Input: part model. Units: mm. Frame: model coordinates. A direction names the side the tool comes from. Give positions to 0.01 mm unless a question says otherwise; leave off trailing zeros. Loops run counter-clockwise (first coordinate to the right, second up) from the corner with the lowest first, then second, coordinate; pieces in that order, holes last. Notation, with made-up numbers: (-24.5, 88) - (-0.5, 88) arc R13 cw to (-0.5, 92) - close; hole circle Ø6 at (-4.5, 54). An arc over 180 degrees is marked (long way). One line per item, written item: value.
Autodesk Inventor part; units mm, degrees
ref_plane "YZ Plane" through (0, 0, 0) normal (1, 0, 0) x (0, 1, 0)
ref_plane "XZ Plane" through (0, 0, 0) normal (0, 1, 0) x (-1, 0, 0)
ref_plane "XY Plane" through (0, 0, 0) normal (0, 0, 1) x (1, 0, 0)
sketch "スケッチ1" plane through (0, 0, 0) normal (0, 0, 1) x (1, 0, 0)
  line L0 (62.5, -15) -> (-62.5, -15)
  line L1 (-62.5, -15) -> (-62.5, 15)
  line L2 (-62.5, 15) -> (62.5, 15)
  line L3 (62.5, 15) -> (62.5, -15)
  line L4 (62.5, -15) -> (-62.5, 15) construction
  line L5 (-62.5, -15) -> (62.5, 15) construction
  point P0 (0, 0)
  dimension "d0" = 30
  dimension "d1" = 125
extrude "押し出し1" add sketch "スケッチ1" along normal blind 34
sketch "スケッチ2" plane through (-62.5, 15, 0) normal (0, 1, 0) x (1, 0, 0)
  line L0 (125, 0) -> (95, 0)
  line L1 (95, 0) -> (95, -6)
  line L2 (95, -6) -> (125, -6)
  line L3 (125, -6) -> (125, 0)
  point P0 (62.5, 0)
  dimension "d4" = 30
  dimension "d5" = 6
extrude "押し出し2" cut sketch "スケッチ2" against normal blind 34
sketch "スケッチ3" plane through (-62.5, 15, 34) normal (0, 1, 0) x (1, 0, 0)
  line L0 (0, 0) -> (125, 0)
  line L1 (90, 0) -> (5, 0)
  line L2 (5, 0) -> (5, 21)
  line L3 (5, 21) -> (90, 21)
  line L4 (90, 21) -> (90, 0)
  line L5 (0, 34) -> (0, 0)
  line L6 (95, 28) -> (95, 34)
  line L7 (95, 34) -> (0, 34)
  point P0 (62.5, 34)
  point P1 (5, 0)
  dimension "d8" = 5
  dimension "d9" = 5
  dimension "d10" = 13
extrude "押し出し3" cut sketch "スケッチ3" against normal blind 34
sketch "スケッチ4" plane through (-62.5, 15, 34) normal (0, 1, 0) x (1, 0, 0)
  line L0 (90, 21) -> (90, 0)
  line L1 (125, 0) -> (90, 0)
  line L2 (125, 28) -> (125, 0)
  line L3 (125, 28) -> (95, 28)
  line L4 (95, 28) -> (95, 34)
  line L5 (95, 34) -> (0, 34)
  line L6 (0, 34) -> (0, 0)
  line L7 (5, 0) -> (0, 0)
  line L8 (5, 0) -> (5, 21)
  line L9 (5, 21) -> (90, 21)
  line L10 (5, 0) -> (5, 21)
  line L11 (5, 0) -> (0, 0)
  line L12 (0, 0) -> (0, 6)
  line L13 (0, 6) -> (5, 6)
  line L14 (5, 6) -> (5, 0)
  point P0 (62.5, 34)
  point P1 (5, 6)
  dimension "d13" = 28
extrude "押し出し4" cut sketch "スケッチ4" against normal blind 34 contours L8 L7 L6 L13
sketch "スケッチ5" plane through (0, 0, 0) normal (0, 0, -1) x (-1, 0, 0)
  line L0 (-12.5, 8.5) -> (42.5, 8.5)
  line L1 (42.5, 8.5) -> (42.5, -8.5)
  line L2 (42.5, -8.5) -> (-12.5, -8.5)
  line L3 (-12.5, -8.5) -> (-12.5, 8.5)
  line L4 (-32.5, 15) -> (-32.5, -15)
  line L5 (62.5, 15) -> (62.5, -15)
  point P0 (0, 0)
  dimension "d17" = 20
  dimension "d18" = 55
  dimension "d26" = 17
  dimension "d27" = 8.5
hole "穴1" at (12.5, 8.5, 0) at (12.5, -8.5, 0) at (-42.5, -8.5, 0) at (-42.5, 8.5, 0) direction (0, 0, 1) diameter 3.3 depth 23
sketch "スケッチ6" plane through (-57.5, 15, 13) normal (0, 0, 1) x (1, 0, 0)
  line L0 (85, -2) -> (0, -2)
  line L1 (0, -2) -> (0, -28)
  line L2 (0, -28) -> (85, -28)
  line L3 (85, -28) -> (85, -2)
  line L4 (0, 0) -> (85, 0)
  line L5 (85, -30) -> (0, -30)
  point P0 (57.5, -15)
  dimension "d28" = 2
  dimension "d29" = 2
extrude "押し出し5" cut sketch "スケッチ6" against normal blind 7.5
sketch "スケッチ7" plane through (-57.5, 15, 5.5) normal (0, 0, 1) x (1, 0, 0)
  circle A0 centre (15, -23.5) radius 1.65
  circle A1 centre (70, -6.5) radius 1.65
  circle A2 centre (70, -23.5) radius 1.65
  circle A3 centre (15, -6.5) radius 1.65
  line L0 (85, -2) -> (85, -28)
  line L1 (0, -2) -> (85, -2)
  line L2 (0, -28) -> (0, -2)
  line L3 (85, -28) -> (0, -28)
  point P0 (57.5, -15)
hole "穴2" at (12.5, 8.5, 5.5) at (-42.5, 8.5, 5.5) at (-42.5, -8.5, 5.5) at (12.5, -8.5, 5.5) direction (0, 0, -1) diameter 3.3 depth 23 counterbore diameter 6.5 counterbore depth 3
sketch "スケッチ8" plane through (0, 0, 34) normal (0, 0, 1) x (1, 0, 0)
  line L0 (62.5, 15) -> (32.5, 15)
  line L1 (62.5, -15) -> (62.5, 15)
  line L2 (32.5, 15) -> (62.5, 15)
  line L3 (62.5, 15) -> (62.5, 14)
  line L4 (62.5, 14) -> (32.5, 14)
  line L5 (32.5, 14) -> (32.5, 15)
  line L6 (62.5, -15) -> (32.5, -15)
  line L7 (32.5, -15) -> (32.5, -14)
  line L8 (32.5, -14) -> (62.5, -14)
  line L9 (62.5, -14) -> (62.5, -15)
  point P0 (0, 0)
  dimension "d39" = 28
  dimension "d40" = 14
extrude "押し出し6" cut sketch "スケッチ8" against normal through all
chamfer "面取り1" distance 2 angle 45 4 edges at (47.5, 14, 34) (47.5, -14, 34) (47.5, 14, 6) (47.5, -14, 6)
sketch "スケッチ9" plane through (-62.5, -15, 0) normal (-1, 0, 0) x (0, 0, 1)
  line L0 (28, 0) -> (28, 30)
  line L1 (0, 30) -> (28, 30)
  line L2 (0, 30) -> (0, 0)
  line L3 (0, 0) -> (28, 0)
  circle A0 centre (20, 15) radius 3
  point P0 (0, 15)
  dimension "d46" = 20
  dimension "d47" = 6
extrude "押し出し7" add sketch "スケッチ9" against normal up to surface (90 mm away) contours A0
properties part number "Linear_Unit_A"
Item 1: Section B-B, the plane y = 8.5. Output: boundary loops of the cut face in (x, z), and give its area (3 significant figures).
Verdict:
outline: (-62.5, 0) - (-44.15, 0) - (-44.15, 2.5) - (-45.75, 2.5) - (-45.75, 5.5) - (-57.5, 5.5) - (-57.5, 28) - (-62.5, 28) - close; (-40.85, 0) - (10.85, 0) - (10.85, 2.5) - (9.25, 2.5) - (9.25, 5.5) - (-39.25, 5.5) - (-39.25, 2.5) - (-40.85, 2.5) - close; (14.15, 0) - (32.5, 0) - (32.5, 6) - (62.5, 6) - (62.5, 34) - (27.5, 34) - (27.5, 5.5) - (15.75, 5.5) - (15.75, 2.5) - (14.15, 2.5) - close
area: 1,560 mm^2
Item 2: Access query for faces 1 (the face through (10.303, 10.895, 3.979)), 2 (the face through (48, 13, 7)), 3 (the face through (-16, -14, 13)). Directions: +Z, -Z, +X, -X, +Y, -Y. A direction counts if a zero-diameter tool reaches every point of the face in a straight line with its end or side. Return the directions, or none.
Verdict:
face 1: +Z
face 2: -Z, +X, +Y
face 3: +Z, +Y, -Y
Item 3: Pin query (flat end, axial travel): P1, Ø1, axis at x = 20, z = 20.5, coming from the -Y side; P2, Ø4, axis at x = -42.5, y = 8.5, coming from the +Z side; P3, Ø8, axis at x = 37.5, y = -3.5, coming from the -Z side. Return the tip coordinate at first contact, or that it passes through.
Verdict:
P1: stops at y = -3
P2: stops at z = 2.5
P3: stops at z = 6
Item 4: Material intervals for L1, parallel to X at y = -8.5, z = 4.1; L2, parallel to Y at x = -42.5, z = 1.4; L3, parallel to Y at x = 12.5, z = 4.45, sorted ascending.
Verdict:
L1: x = -62.5 to -45.75, -39.25 to 9.25, 15.75 to 32.5
L2: y = -15 to -10.15, -6.85 to 6.85, 10.15 to 15
L3: y = -15 to -11.75, -5.25 to 5.25, 11.75 to 15
Item 5: Section C-C, the plane z = 20. Output: boundary loops of the cut face in (x, y), and give its area (3 significant figures).
Verdict:
outline: (-62.5, -15) - (-57.5, -15) - (-57.5, -3) - (27.5, -3) - (27.5, -15) - (32.5, -15) - (32.5, -14) - (62.5, -14) - (62.5, 14) - (32.5, 14) - (32.5, 15) - (27.5, 15) - (27.5, 3) - (-57.5, 3) - (-57.5, 15) - (-62.5, 15) - close
area: 1,650 mm^2
Item 6: Section A-A, the plane x = -36.5. Output: boundary loops of the cut face in (y, z), and give its area (3 significant figures).
Verdict:
outline: (-15, 0) - (15, 0) - (15, 13) - (13, 13) - (13, 5.5) - (-13, 5.5) - (-13, 13) - (-15, 13) - close; circle Ø6 at (0, 20)
area: 223 mm^2
Item 7: Section D-D, the plane x = 12.5. Output: boundary loops of the cut face in (y, z), and give its area (3 significant figures).
Verdict:
outline: (-15, 0) - (-10.15, 0) - (-10.15, 2.5) - (-11.75, 2.5) - (-11.75, 5.5) - (-13, 5.5) - (-13, 13) - (-15, 13) - close; (-6.85, 0) - (6.85, 0) - (6.85, 2.5) - (5.25, 2.5) - (5.25, 5.5) - (-5.25, 5.5) - (-5.25, 2.5) - (-6.85, 2.5) - close; circle Ø6 at (0, 20); (10.15, 0) - (15, 0) - (15, 13) - (13, 13) - (13, 5.5) - (11.75, 5.5) - (11.75, 2.5) - (10.15, 2.5) - close
area: 168 mm^2
Item 8: Draft query along Y for faces 4 (the face through (27.5, 4, 20)), 5 (the face through (-41, 7, 2.5)), 6 (the face through (47, 0, 6)), 7 (the face through (48, 14, 20)). Return one class per face: pulls with the +Y half, pulls with the -Y half, needs draft (parallel to the pull), parting line crosses it, or undercut.
Verdict:
face 4: undercut
face 5: undercut
face 6: needs draft
face 7: pulls with the +Y half
